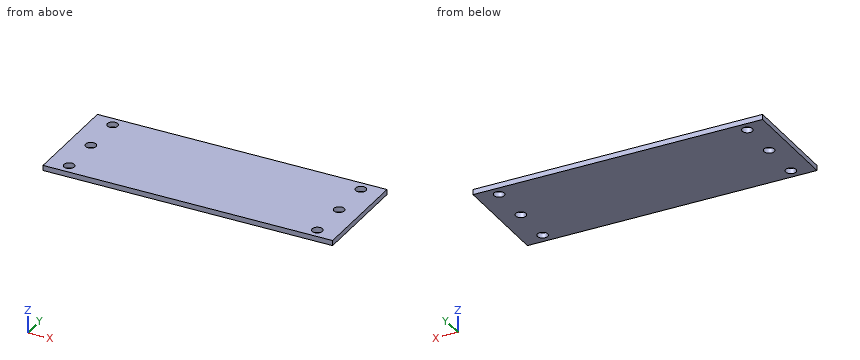
Autodesk Inventor part; units mm, degrees
ref_plane "YZ Plane" through (0, 0, 0) normal (1, 0, 0) x (0, 1, 0)
ref_plane "XZ Plane" through (0, 0, 0) normal (0, 1, 0) x (-1, 0, 0)
ref_plane "XY Plane" through (0, 0, 0) normal (0, 0, 1) x (1, 0, 0)
sketch "Sketch1" plane through (0, 0, 0) normal (0, 0, 1) x (1, 0, 0)
  line L0 (-0.2558, -58.1023) -> (177.5442, -58.1023)
  line L1 (177.5442, -58.1023) -> (177.5442, 5.3977)
  line L2 (177.5442, 5.3977) -> (-0.2558, 5.3977)
  line L3 (-0.2558, 5.3977) -> (-0.2558, -58.1023)
  point P0 (0, 0)
  dimension "d0" = 177.8
  dimension "d1" = 63.5
extrude "Extrusion1" add sketch "Sketch1" along normal blind 3.175
sketch "Sketch3" plane through (0, 0, 3.175) normal (0, 0, 1) x (1, 0, 0)
  line L0 (-0.2558, 5.3977) -> (-0.2558, -58.1023)
  line L1 (177.5442, 5.3977) -> (-0.2558, 5.3977)
  line L2 (-0.2558, -58.1023) -> (177.5442, -58.1023)
  line L3 (177.5442, -58.1023) -> (177.5442, 5.3977)
  point P0 (0, 0)
  point P1 (12.4442, -0.9523)
  point P2 (12.4442, -26.3523)
  point P3 (12.4442, -51.7523)
  point P4 (164.8442, -0.9523)
  point P5 (164.8442, -26.3523)
  point P6 (164.8442, -51.7523)
  dimension "d22" = 25.4
  dimension "d23" = 25.4
  dimension "d26" = 12.7
  dimension "d27" = 12.7
  dimension "d28" = 12.7
  dimension "d29" = 6.35
  dimension "d30" = 6.35
  dimension "d33" = 6.35
  dimension "d34" = 25.4
  dimension "d35" = 25.4
  dimension "d36" = 12.7
hole "Hole2" at (12.4442, -0.9523, 3.175) at (12.4442, -26.3523, 3.175) at (12.4442, -51.7523, 3.175) at (164.8442, -0.9523, 3.175) at (164.8442, -26.3523, 3.175) at (164.8442, -51.7523, 3.175) direction (0, 0, -1) diameter 6.35 end through all
properties part number "base and top plate real"
Work out the finished part from the listing and answer in its coordinate system (mm). Give positions to 0.01 mm unless a question says otherwise; leave off trailing zeros. Loops run counter-clockwise (first coordinate to the right, second up) from the corner with the lowest first, then second, coordinate; pieces in that order, holes last. Notation, with made-up numbers: (45, 67) -> (99, 67) arc R21 ccw to (99, 80) -> close; hole circle Ø1 at (25, 15.25). An arc over 180 degrees is marked (long way). Put each result on its own line as item: value. Start each with the question number.
Item 1: The part is cut by section A-A (y = -51.5). Give the vertices of the cut face in (x, z) (3 decimals).
Item 2: This flat-tipped pin is pushed along its axis until it touches: P1, Ø1, axis at x = 102.5, y = -40, coming from the -Z side. Where does it stop, or does it pass through?
Item 3: The part is cut by section C-C (y = -0.5). Give the vertices of the cut face in (x, z) (3 decimals).
Item 4: The part is cut by section B-B (z = 1.3). Give the vertices of the cut face in (x, y) (3 decimals), then the cut area to 3 significant figures.
Item 5: Find the intervals of material crossed by L1, parallel to X at y = -28.5, z = 1.9, in increasing order. Write a range as [from, to].
Answers below:
1. outline: (-0.256, 0) -> (9.279, 0) -> (9.279, 3.175) -> (-0.256, 3.175) -> close; (15.609, 0) -> (161.679, 0) -> (161.679, 3.175) -> (15.609, 3.175) -> close; (168.009, 0) -> (177.544, 0) -> (177.544, 3.175) -> (168.009, 3.175) -> close
2. P1: z = 0
3. outline: (-0.256, 0) -> (9.302, 0) -> (9.302, 3.175) -> (-0.256, 3.175) -> close; (15.587, 0) -> (161.702, 0) -> (161.702, 3.175) -> (15.587, 3.175) -> close; (167.987, 0) -> (177.544, 0) -> (177.544, 3.175) -> (167.987, 3.175) -> close
4. outline: (-0.256, -58.102) -> (177.544, -58.102) -> (177.544, 5.398) -> (-0.256, 5.398) -> close; hole circle Ø6.35 at (12.444, -51.752); hole circle Ø6.35 at (12.444, -26.352); hole circle Ø6.35 at (12.444, -0.952); hole circle Ø6.35 at (164.844, -51.752); hole circle Ø6.35 at (164.844, -26.352); hole circle Ø6.35 at (164.844, -0.952)
4. area: 11,100 mm2
5. L1: [-0.26, 10.11], [14.78, 162.51], [167.18, 177.54]
